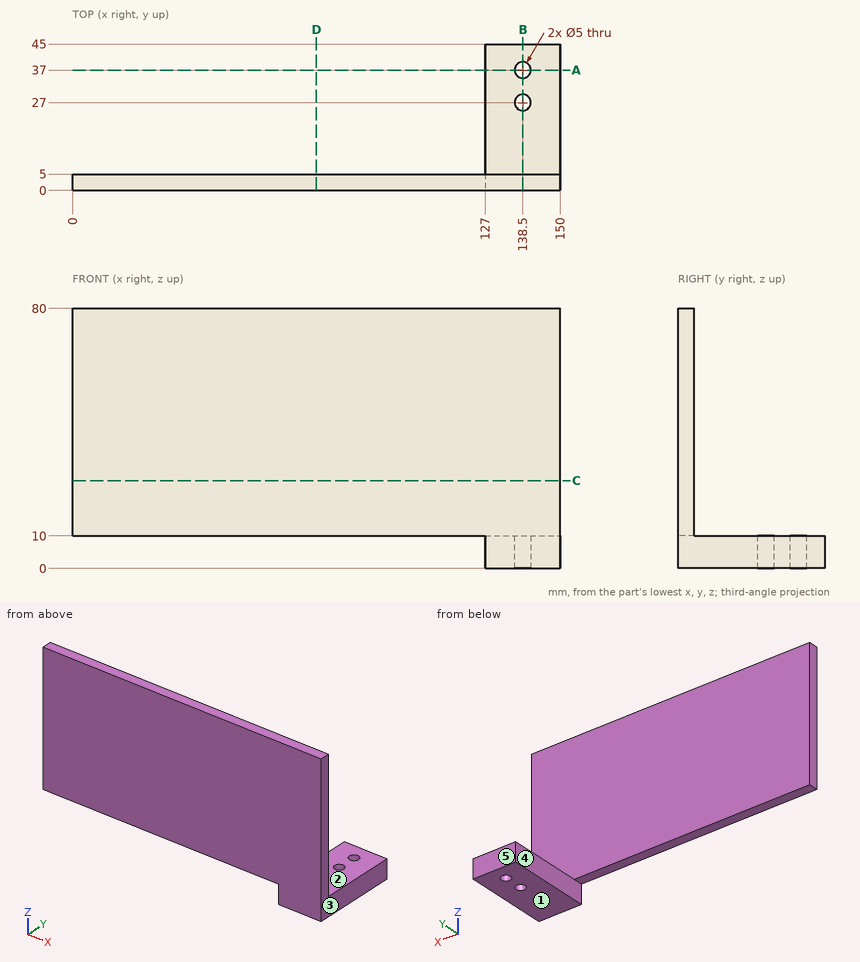
The figure shows three views and two pictorial views of one solid part (mm, origin at its lowest corner). Answer the questions. A direction names the side the tool comes from. Coordinates: 2 decimals unless noted, no trailing zeros. Loops run counter-clockwise (first coordinate to the right, second up) from the corner with the lowest first, then second, coordinate; pieces in that order, holes last. Notation, with made-up numbers: (59, 23) -> (74, 23) arc R26 cw to (74, 40) -> close; hole circle Ø1 at (46, 88). An arc over 180 degrees is marked (long way). Write item = value, one per line. Start each with the question number.
1) A cutting plane is placed at C-C (z = 27). Give the vertices of the cut face in (x, y).
2) The mould has two halves that part along X. Classify the marked faces 3, 4 and 5: released by +X, released by -X, zero draft, split by the parting line, or undercut.
3) Straight lines are drawn through the part: line 1 (Y direction, x = 138.5, z = 8.25); line 2 (Y direction, x = 138, z = 7); line 3 (Y direction, x = 96.5, z = 42). For each, find the intervals that lie inside material, in ascending order. Write a range as from..to.
4) Given pin 1 Ø6.5 at (x, y) = (138.5, 37) entering from -Z; pin 2 Ø12 at (x, z) = (17.5, 47) entering from +Y; pin 3 Ø11.5 at (x, y) = (141, 28) entering from +Z; pin 4 Ø4 at (x, y) = (40.5, 3) entering from -Z, each flat-ended and moving along its own axis, determine where each tip first touches the part or whether it passes through.
5) A cutting plane is placed at B-B (x = 138.5). Give the vertices of the cut face in (y, z).
6) A cutting plane is placed at A-A (y = 37). Give the vertices of the cut face in (x, z).
7) A tool of negligible diameter and unlimited length cuts with its end or side. For the marked faces 1 and 2, from which of +Z, -Z, +X, -X, +Y, -Y can it reach the whole face along a straight path? Write none if from no direction.
8) A cutting plane is placed at D-D (x = 75). Give the vertices of the cut face in (y, z).
Responses:
q1.outline = (0, 0) -> (150, 0) -> (150, 5) -> (0, 5) -> close
q2.face_3 = released by +X
q2.face_4 = released by -X
q2.face_5 = zero draft
q3.line_1 = 0..24.5, 29.5..34.5, 39.5..45
q3.line_2 = 0..24.55, 29.45..34.55, 39.45..45
q3.line_3 = 0..5
q4.pin_1 = 0
q4.pin_2 = 5
q4.pin_3 = 10
q4.pin_4 = 10
q5.outline = (0, 0) -> (24.5, 0) -> (24.5, 10) -> (5, 10) -> (5, 80) -> (0, 80) -> close; (29.5, 0) -> (34.5, 0) -> (34.5, 10) -> (29.5, 10) -> close; (39.5, 0) -> (45, 0) -> (45, 10) -> (39.5, 10) -> close
q6.outline = (127, 0) -> (136, 0) -> (136, 10) -> (127, 10) -> close; (141, 0) -> (150, 0) -> (150, 10) -> (141, 10) -> close
q7.face_1 = -Z, +X, -X, +Y, -Y
q7.face_2 = +Z, +X, -X, +Y
q8.outline = (0, 10) -> (5, 10) -> (5, 80) -> (0, 80) -> close
